The listing builds one solid part. Answer for the finished solid, in the listing's coordinates (mm). A direction names the side the tool comes from. Coordinates: 2 decimals unless noted, no trailing zeros. Loops run counter-clockwise (first coordinate to the right, second up) from the corner with the lowest first, then second, coordinate; pieces in that order, holes last. Notation, with made-up numbers: (57, 28.5) -> (104, 28.5) arc R32 cw to (104, 64.5) -> close; hole circle Ø3 at (-3.75, 14). An arc over 180 degrees is marked (long way). Answer in a Markdown table with one row per item.
```python
from build123d import *

# Parameters (mm, degrees)
SKETCH1_W               = 50
SKETCH1_H               = 40
BOSS_EXTRUDE1_DEPTH     = 20
BOSS_EXTRUDE2_START     = -20
SKETCH3_W               = 35
SKETCH3_H               = 4
BOSS_EXTRUDE2_DEPTH     = 20
SKETCH4_R               = 2.25
CUT_EXTRUDE1_DEPTH      = 5
LPATTERN1_COUNT         = 3
LPATTERN1_PITCH         = 10
MIRROR1_COPY_1_SKETCH_R = 2.25
MIRROR1_COPY_1_DEPTH    = 5
MIRROR1_COPY_2_SKETCH_R = 2.25
MIRROR1_COPY_2_DEPTH    = 5
CUT_EXTRUDE2_DEPTH      = 75.833147735
CUT_EXTRUDE2_DEPTH_BACK = 75.833147735
SKETCH6_W               = 38
SKETCH6_H               = 28
CUT_EXTRUDE3_DEPTH      = 15
CUT_EXTRUDE4_DEPTH      = 66
FILLET1_R               = 2.5
FILLET2_R               = 4
FILLET3_R               = 4


with BuildPart() as part:
    # Sketch1 → Boss-Extrude1 (new body)
    with BuildSketch(Plane(origin=(0, 0, 0), x_dir=(1, 0, 0), z_dir=(0, 1, 0))):
        Rectangle(SKETCH1_W, SKETCH1_H)
    extrude(amount=BOSS_EXTRUDE1_DEPTH)

    # Sketch3 → Boss-Extrude2 (add)
    with BuildSketch(Plane(origin=(0, 20, 0), x_dir=(1, 0, 0), z_dir=(0, 1, 0)).offset(BOSS_EXTRUDE2_START)):
        with Locations((42.5, -4)):
            Rectangle(SKETCH3_W, SKETCH3_H)
    boss_extrude2 = extrude(amount=BOSS_EXTRUDE2_DEPTH)

    # Sketch4 → Cut-Extrude1 (cut)
    with BuildSketch(Plane.XY.offset(6)):
        with Locations((55, 12.5)):
            Circle(SKETCH4_R)
    cut_extrude1 = extrude(amount=-CUT_EXTRUDE1_DEPTH, mode=Mode.SUBTRACT)

    # LPattern1: Cut-Extrude1 ×3
    with Locations(*[(-i * LPATTERN1_PITCH, 0, 0) for i in range(1, LPATTERN1_COUNT)]):
        add(cut_extrude1, mode=Mode.SUBTRACT)

    # Mirror1: Boss-Extrude2, Cut-Extrude1 across plane
    add(boss_extrude2.mirror(Plane.XY))
    add(cut_extrude1.mirror(Plane.XY), mode=Mode.SUBTRACT)

    # Mirror1 copy 1 sketch → Mirror1 copy 1 (cut)
    with BuildSketch(Plane(origin=(-10, 0, -6), x_dir=(1, 0, 0), z_dir=(0, 0, -1))):
        with Locations((55, -12.5)):
            Circle(MIRROR1_COPY_1_SKETCH_R)
    extrude(amount=-MIRROR1_COPY_1_DEPTH, mode=Mode.SUBTRACT)

    # Mirror1 copy 2 sketch → Mirror1 copy 2 (cut)
    with BuildSketch(Plane(origin=(-20, 0, -6), x_dir=(1, 0, 0), z_dir=(0, 0, -1))):
        with Locations((55, -12.5)):
            Circle(MIRROR1_COPY_2_SKETCH_R)
    extrude(amount=-MIRROR1_COPY_2_DEPTH, mode=Mode.SUBTRACT)

    # Sketch5 → Cut-Extrude2 (cut, two sides)
    with BuildSketch(Plane.XY.offset(20)) as cut_extrude2_sk:
        Polygon((23, 20), (-25, 2), (-25, 20), align=None)
    extrude(amount=CUT_EXTRUDE2_DEPTH, mode=Mode.SUBTRACT)
    extrude(cut_extrude2_sk.sketch, amount=-CUT_EXTRUDE2_DEPTH_BACK, mode=Mode.SUBTRACT)

    # Sketch6 → Cut-Extrude3 (cut)
    with BuildSketch(Plane(origin=(0, 20, 0), x_dir=(1, 0, 0), z_dir=(0, 1, 0))):
        Rectangle(SKETCH6_W, SKETCH6_H)
    extrude(amount=-CUT_EXTRUDE3_DEPTH, mode=Mode.SUBTRACT)

    # Sketch7 → Cut-Extrude4 (cut, symmetric)
    with BuildSketch(Plane(origin=(0, 5, 0), x_dir=(1, 0, 0), z_dir=(0, 1, 0))):
        with BuildLine():
            Line((13.25, 8), (13.25, -8))
            ThreePointArc((13.25, -8), (10, -11.25), (6.75, -8))
            Line((6.75, -8), (6.75, 8))
            ThreePointArc((6.75, 8), (10, 11.25), (13.25, 8))
        make_face()
    cut_extrude4 = extrude(amount=CUT_EXTRUDE4_DEPTH, both=True, mode=Mode.SUBTRACT)

    # Mirror2: Cut-Extrude4 across plane
    add(cut_extrude4.mirror(Plane(origin=(0, 0, 0), x_dir=(0, 0, 1), z_dir=(1, 0, 0))), mode=Mode.SUBTRACT)

    # Fillet1
    fillet1_edges = [part.edges().sort_by_distance(p)[0] for p in [
        (60, 20, 4),
        (60, 20, -4),
    ]]
    fillet(fillet1_edges, radius=FILLET1_R)

    # Fillet2
    fillet2_edges = [part.edges().sort_by_distance(p)[0] for p in [
        (25, 10, 6),
        (25, 10, -6),
    ]]
    fillet(fillet2_edges, radius=FILLET2_R)

    # Fillet3
    fillet3_edges = [part.edges().sort_by_distance(p)[0] for p in [
        (-25, 1, -20),
        (-25, 1, 20),
        (25, 10, -20),
        (25, 10, 20),
    ]]
    fillet(fillet3_edges, radius=FILLET3_R)


solid = part.part
```
Item 1: Find the intervals of material crossed by probe 1 along X at (y, z) = (12.5, -3.25); probe 2 along Z at (x, y) = (5.5, 12); probe 3 along Z at (x, y) = (54.5, 18.25), in increasing order.
Findings below:
| item | result |
|---|---|
| probe 1 | x = 19 to 32.75, 37.25 to 42.75, 47.25 to 52.75, 57.25 to 60 |
| probe 2 | z = -20 to -14, 14 to 20 |
| probe 3 | z = -6 to -2, 2 to 6 |
Item 2: A cutting plane is placed at D-D, the plane z = 9. Determine the outline of the cut face in (x, y).
Findings below:
| item | result |
|---|---|
| outline | (-25, 0) -> (-13.09, 0) -> (-13.09, 5) -> (-17, 5) -> (-25, 2) -> close; (-6.91, 0) -> (6.91, 0) -> (6.91, 5) -> (-6.91, 5) -> close; (13.09, 0) -> (25.13, 0) -> (25.13, 20) -> (23, 20) -> (19, 18.5) -> (19, 5) -> (13.09, 5) -> close |
Item 3: Flat-ended cylindrical pins translate along their axes: pin 1 Ø10 at (x, z) = (44, -3.5) entering from -Y; pin 2 Ø6 at (x, y) = (35, 12.5) entering from +Z; pin 3 Ø7 at (y, z) = (9.5, 7) entering from -X; pin 4 Ø4 at (x, y) = (55, 12.5) entering from +Z. Find the tip coordinate at first contact, or state that the pin passes through.
Findings below:
| item | result |
|---|---|
| pin 1 | stops at y = 0 |
| pin 2 | stops at z = 6 |
| pin 3 | stops at x = 19 |
| pin 4 | passes through |
Item 4: A cutting plane is placed at C-C, the plane x = -10. Determine the outline of the cut face in (y, z) (3 decimals).
Findings below:
| item | result |
|---|---|
| outline | (0, -20) -> (7.625, -20) -> (7.625, -14) -> (5, -14) -> (5, -11.25) -> (0, -11.25) -> close; (0, 11.25) -> (5, 11.25) -> (5, 14) -> (7.625, 14) -> (7.625, 20) -> (0, 20) -> close |
Item 5: A cutting plane is placed at A-A, the plane z = -3. Determine the outline of the cut face in (x, y), plus the area to 3 significant figures.
Findings below:
| item | result |
|---|---|
| outline | (-25, 0) -> (-13.25, 0) -> (-13.25, 5) -> (-17, 5) -> (-25, 2) -> close; (-6.75, 0) -> (6.75, 0) -> (6.75, 5) -> (-6.75, 5) -> close; (13.25, 0) -> (60, 0) -> (60, 17.5) arc R2.5 ccw to (57.5, 20) -> (23, 20) -> (19, 18.5) -> (19, 5) -> (13.25, 5) -> close; hole circle Ø4.5 at (35, 12.5); hole circle Ø4.5 at (45, 12.5); hole circle Ø4.5 at (55, 12.5) |
| area | 911 mm2 |
Item 6: Determine the mould class of faces 5 (the face through (42, 10, -2)), 6 (the face through (6.75, 3, 0)), 7 (the face through (26.203, 10.14, 7.141)) for opening direction X: +X half, -X half, draft (parallel to the pull), parting line (faces both ways), or undercut.
Findings below:
| item | result |
|---|---|
| face 5 | draft |
| face 6 | undercut |
| face 7 | +X half |
Item 7: A tool of negligible diameter and unlimited length cuts with its end or side. For faces 1 (the face through (44, 10, -6)), 2 (the face through (-9.93, 2.54, -11.25)), 3 (the face through (25, 10, 0)), 4 (the face through (44, 10, 6)), from which of +Z, -Z, +X, -X, +Y, -Y can it reach the whole face along a straight path? Write none if from no direction.
Findings below:
| item | result |
|---|---|
| face 1 | -Z, +X, +Y, -Y |
| face 2 | +Y, -Y |
| face 3 | +X, +Y, -Y |
| face 4 | +Z, +X, +Y, -Y |
Item 8: A cutting plane is placed at B-B, the plane x = 35. Determine the outline of the cut face in (y, z).
Findings below:
| item | result |
|---|---|
| outline | (0, -6) -> (10.25, -6) -> (10.25, -2) -> (0, -2) -> close; (0, 2) -> (10.25, 2) -> (10.25, 6) -> (0, 6) -> close; (14.75, -6) -> (20, -6) -> (20, -2) -> (14.75, -2) -> close; (14.75, 2) -> (20, 2) -> (20, 6) -> (14.75, 6) -> close |
